Build history of the part. All positions in model axes, mm. Round coordinates to 2 decimals unless told otherwise and drop trailing zeros.
from build123d import *

# Parameters (mm, degrees)
F1_DEPTH = 3.175


with BuildPart() as f1:
    # F0 (on Front) → F1 (new body)
    with BuildSketch(Plane.XZ):
        Polygon((0, 20.0025), (0, 0), (77.9907, 0), (77.9907, 40.005), (0, 40.005), align=None)
        with BuildLine():
            ThreePointArc((7.4944, 20.0025), (5.9944, 18.5025), (4.4944, 20.0025))
            ThreePointArc((4.4944, 20.0025), (5.9944, 21.5025), (7.4944, 20.0025))
        make_face(mode=Mode.SUBTRACT)
        with BuildLine():
            ThreePointArc((31.9913, 18.5025), (30.93064, 18.94184), (30.4913, 20.0025))
            ThreePointArc((30.4913, 20.0025), (31.9913, 21.5025), (33.4913, 20.0025))
            ThreePointArc((33.4913, 20.0025), (33.05196, 18.94184), (31.9913, 18.5025))
        make_face(mode=Mode.SUBTRACT)
        with BuildLine():
            ThreePointArc((59.4882, 20.0025), (57.9882, 18.5025), (56.4882, 20.0025))
            ThreePointArc((56.4882, 20.0025), (57.9882, 21.5025), (59.4882, 20.0025))
        make_face(mode=Mode.SUBTRACT)
    extrude(amount=F1_DEPTH)


solid = f1.part
1) Pin check, flat tips, straight feed: pin 1 Ø3.5 at (x, z) = (57.99, 20) entering from -Y (3 decimals); pin 2 Ø2.5 at (x, z) = (5.99, 20) entering from +Y. Stop position of each tip, or through.
Results:
pin 1: stops at y = -3.175
pin 2: passes through
2) Wall check: L1, parallel to X at y = -2.75, z = 19.5. Give the ranges that are in metal, low to high.
Results:
L1: x = 0 to 4.58, 7.41 to 30.58, 33.4 to 56.57, 59.4 to 77.99
3) Mould opens along Z. For faces 1 (the cylindrical face through (59.09, -1.57, 21.02)), 2 (the flat face through (77.991, -2, 20)), 3 (the flat face through (38, -2, 0)) say: released by +Z, released by -Z, zero draft, split by the parting line, or undercut.
Results:
face 1: undercut
face 2: zero draft
face 3: released by -Z
